Autodesk Inventor part; units mm, degrees
ref_plane "YZ Plane" through (0, 0, 0) normal (1, 0, 0) x (0, 1, 0)
ref_plane "XZ Plane" through (0, 0, 0) normal (0, 1, 0) x (-1, 0, 0)
ref_plane "XY Plane" through (0, 0, 0) normal (0, 0, 1) x (1, 0, 0)
sketch "Sketch1" plane through (0, 0, 0) normal (0, 1, 0) x (-1, 0, 0)
  line L0 (-50, 50) -> (50, 50)
  line L1 (50, 50) -> (50, -50)
  line L2 (50, -50) -> (-50, -50)
  line L3 (-50, -50) -> (-50, 50)
  line L4 (-50, 50) -> (50, -50) construction
  line L5 (50, 50) -> (-50, -50) construction
  circle A0 centre (46.444, 46.444) radius 1.5875
  circle A1 centre (46.444, -46.444) radius 1.5875
  circle A2 centre (-46.444, -46.444) radius 1.5875
  circle A3 centre (-46.444, 46.444) radius 1.5875
  point P0 (0, 0)
  dimension "d0" = 100
  dimension "d1" = 100
  dimension "d2" = 3.175
  dimension "d3" = 3.175
  dimension "d4" = 3.175
  dimension "d5" = 3.175
  dimension "d6" = 3.556
  dimension "d7" = 3.556
  dimension "d8" = 3.556
  dimension "d9" = 3.556
extrude "Extrusion1" add sketch "Sketch1" along normal blind 1.5875
sketch "Sketch2" plane through (0, 1.5875, 0) normal (0, 1, 0) x (1, 0, 0)
  line L0 (-21.12, -50) -> (24.6, -50)
  line L1 (24.6, -50) -> (24.6, -47.46)
  line L2 (24.6, -47.46) -> (-21.12, -47.46)
  line L3 (-21.12, -47.46) -> (-21.12, -50)
  line L4 (50, 50) -> (-50, 50)
  line L5 (-17.31, 50) -> (18.25, 50)
  line L6 (18.25, 50) -> (18.25, 47.46)
  line L7 (18.25, 47.46) -> (-17.31, 47.46)
  line L8 (-17.31, 47.46) -> (-17.31, 50)
  line L9 (50, 8.42) -> (47.46, 8.42)
  line L10 (47.46, 8.42) -> (47.46, -9.36)
  line L11 (47.46, -9.36) -> (50, -9.36)
  line L12 (50, -9.36) -> (50, 8.42)
  line L13 (50, -50) -> (50, 50)
  line L14 (-50, -50) -> (50, -50)
  point P0 (0, 0)
  dimension "d12" = 2.54
  dimension "d13" = 2.54
  dimension "d14" = 2.54
  dimension "d15" = 0
  dimension "d16" = 0
  dimension "d17" = 25.4
  dimension "d18" = 45.72
  dimension "d19" = 17.78
  dimension "d20" = 35.56
  dimension "d21" = 40.64
  dimension "d22" = 31.75
extrude "Extrusion2" add sketch "Sketch2" along normal blind 8.509
properties part number "Board"
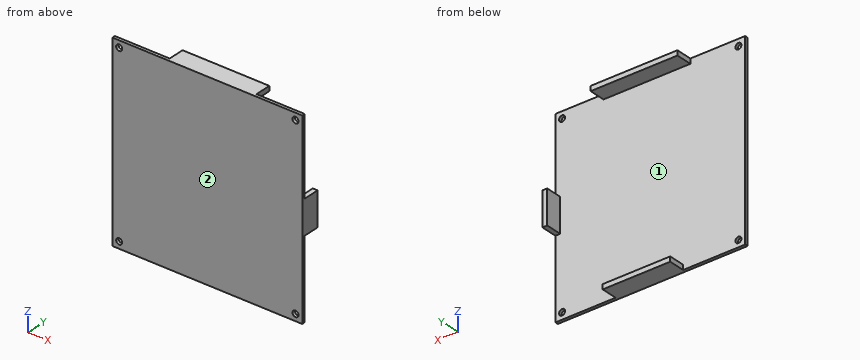
The listing builds one solid part. Answer for the finished solid, in the listing's coordinates (mm). Face numbers are marked on the shaded views. Round coordinates to 2 decimals unless told otherwise and drop trailing zeros. Write each loop counter-clockwise with the first axis right and the second up, starting at its lowest first coordinate (ties: lowest second). Pieces come first, ordered by that corner, then holes. Notation, with made-up numbers: M 54.25,-31.5 L 93.25,-31.5 A28 ccw 93.25,6.5 Z; hole C 70.5,82 d6. An arc over 180 degrees is marked long. Write each question's results on one line, items separated by ' | '. Start each with the question number.
(1) The part is cut by section A-A, the plane y = 8. Write down the section's boundary in (x, z), and give its area (3 significant figures).
(2) Find the intervals of material crossed by line 1 (Z direction, x = -6.5, y = 8.5); line 2 (Y direction, x = -22, z = -36.5); line 3 (Z direction, x = -20, y = 6.75), in increasing order.
(3) The part is cut by section D-D, the plane x = -7. Write down the section's boundary in (y, z), and give its area (3 significant figures).
(4) Each of these flat-tipped pins is pushed along its axis until it touches: P1, Ø2.5, axis at x = 46.444, z = -46.444, coming from the +Y side; P2, Ø0.8, axis at x = 48.5, y = 4, coming from the -Z side; P3, Ø4.5, axis at y = 4, z = 3, coming from the -X side; P4, Ø2, axis at x = 49, y = 7.5, coming from the +Z side. Where does it stop, or does it pass through?
(5) The part is cut by section B-B, the plane x = -18.5. Write down the section's boundary in (y, z).
(6) Determine the mould class of the marked faces 1 and 2 for opening direction Z: +Z half, -Z half, draft (parallel to the pull), parting line (faces both ways), or undercut.
(7) The part is cut by section C-C, the plane z = 0. Write down the section's boundary in (x, y).
Worked answers:
1) outline: M -21.12,47.46 L 24.6,47.46 L 24.6,50 L -21.12,50 Z; M -17.31,-50 L 18.25,-50 L 18.25,-47.46 L -17.31,-47.46 Z; M 47.46,-8.42 L 50,-8.42 L 50,9.36 L 47.46,9.36 Z | area: 252 mm²
2) line 1: z = -50 to -47.46, 47.46 to 50 | line 2: y = 0 to 1.59 | line 3: z = 47.46 to 50
3) outline: M 0,-50 L 10.1,-50 L 10.1,-47.46 L 1.59,-47.46 L 1.59,47.46 L 10.1,47.46 L 10.1,50 L 0,50 Z | area: 202 mm²
4) P1: passes through | P2: stops at z = -8.42 | P3: stops at x = 47.46 | P4: stops at z = 9.36
5) outline: M 0,-50 L 1.59,-50 L 1.59,47.46 L 10.1,47.46 L 10.1,50 L 0,50 Z
6) face 1: undercut | face 2: draft
7) outline: M -50,0 L 50,0 L 50,10.1 L 47.46,10.1 L 47.46,1.59 L -50,1.59 Z
